Check sheet for the modelled part. Datum: model origin and axes. Units: mm. Round coordinates to 2 decimals unless told otherwise and drop trailing zeros. Write each loop counter-clockwise with the first axis right and the second up, starting at its lowest first coordinate (ties: lowest second). Pieces come first, ordered by that corner, then holes. Notation, with made-up numbers: (77.25, 41) -> (113.25, 41) arc R21 cw to (113.25, 70) -> close; hole circle Ø2 at (44.5, 52.5). An arc over 180 degrees is marked (long way). One line per item, written item: value.
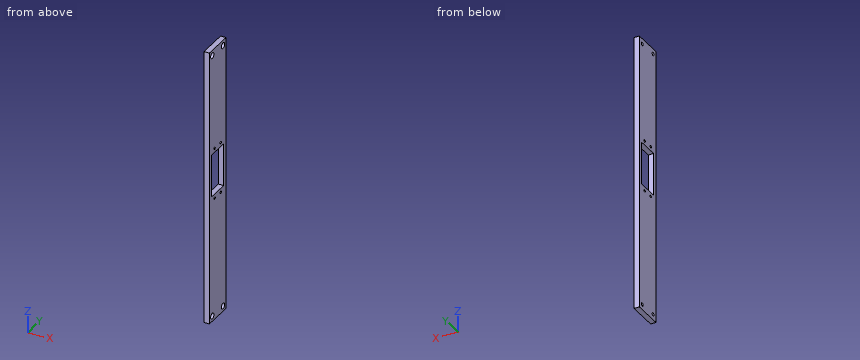
from build123d import *

# Parameters (mm, degrees)
SKETCH1_W                                  = 5
SKETCH1_H                                  = 260.2
BOSS_EXTRUDE1_DEPTH                        = 28
SKETCH2_W                                  = 40.12
SKETCH2_H                                  = 20.12
CUT_EXTRUDE1_DEPTH                         = 134.172857595
SKETCH3_R                                  = 1.125
CUT_EXTRUDE2_DEPTH                         = 134.172857595
SKETCH4_R                                  = 2.75
CUT_EXTRUDE3_DEPTH                         = 3
SKETCH5_R                                  = 1.55
CUT_EXTRUDE4_DEPTH                         = 134.112771739
MIRROR2_AT_THE_SECOND_PLANE_COPY_1_SKETC_R = 2.75
MIRROR2_AT_THE_SECOND_PLANE_COPY_1_DEPTH   = 3
MIRROR2_AT_THE_SECOND_PLANE_COPY_2_SKETC_R = 1.55
MIRROR2_AT_THE_SECOND_PLANE_COPY_2_DEPTH   = 134.112771739


with BuildPart() as part:
    # Sketch1 → Boss-Extrude1 (new body)
    with BuildSketch(Plane(origin=(0, 0, 0), x_dir=(1, 0, 0), z_dir=(0, 1, 0))):
        Rectangle(SKETCH1_W, SKETCH1_H)
    extrude(amount=BOSS_EXTRUDE1_DEPTH)

    # Sketch2 → Cut-Extrude1 (cut, through all)
    with BuildSketch(Plane(origin=(2.5, 0, 0), x_dir=(0, 0, -1), z_dir=(1, 0, 0))):
        with Locations((-10.06, 14)):
            Rectangle(SKETCH2_W, SKETCH2_H)
    extrude(amount=-CUT_EXTRUDE1_DEPTH, mode=Mode.SUBTRACT)

    # Sketch3 → Cut-Extrude2 (cut, through all)
    with BuildSketch(Plane(origin=(2.5, 0, 0), x_dir=(0, 0, -1), z_dir=(1, 0, 0))):
        with Locations((-33.96, 19.1)):
            Circle(SKETCH3_R)
        with Locations((-33.96, 8.9)):
            Circle(SKETCH3_R)
        with Locations((13.84, 19.1)):
            Circle(SKETCH3_R)
        with Locations((13.84, 8.9)):
            Circle(SKETCH3_R)
    extrude(amount=-CUT_EXTRUDE2_DEPTH, mode=Mode.SUBTRACT)

    # Sketch4 → Cut-Extrude3 (cut)
    with BuildSketch(Plane(origin=(2.5, 0, 0), x_dir=(0, 0, -1), z_dir=(1, 0, 0))):
        with Locations((-125.1, 23)):
            Circle(SKETCH4_R)
    cut_extrude3 = extrude(amount=-CUT_EXTRUDE3_DEPTH, mode=Mode.SUBTRACT)

    # Sketch5 → Cut-Extrude4 (cut, through all)
    with BuildSketch(Plane(origin=(-0.5, 0, 0), x_dir=(0, 0, -1), z_dir=(1, 0, 0))):
        with Locations((-125.1, 23)):
            Circle(SKETCH5_R)
    cut_extrude4 = extrude(amount=-CUT_EXTRUDE4_DEPTH, mode=Mode.SUBTRACT)

    # Mirror2: Cut-Extrude3, Cut-Extrude4 across plane
    add(cut_extrude3.mirror(Plane.XY), mode=Mode.SUBTRACT)
    add(cut_extrude4.mirror(Plane.XY), mode=Mode.SUBTRACT)

    # Mirror2 at the second plane: Cut-Extrude3, Cut-Extrude4 across plane
    add(cut_extrude3.mirror(Plane.ZX.offset(14)), mode=Mode.SUBTRACT)
    add(cut_extrude4.mirror(Plane.ZX.offset(14)), mode=Mode.SUBTRACT)

    # Mirror2 at the second plane copy 1 sketc → Mirror2 at the second plane copy 1 (cut)
    with BuildSketch(Plane(origin=(2.5, 28, 0), x_dir=(0, 0, 1), z_dir=(1, 0, 0))):
        with Locations((-125.1, 23)):
            Circle(MIRROR2_AT_THE_SECOND_PLANE_COPY_1_SKETC_R)
    extrude(amount=-MIRROR2_AT_THE_SECOND_PLANE_COPY_1_DEPTH, mode=Mode.SUBTRACT)

    # Mirror2 at the second plane copy 2 sketc → Mirror2 at the second plane copy 2 (cut, through all)
    with BuildSketch(Plane(origin=(-0.5, 28, 0), x_dir=(0, 0, 1), z_dir=(1, 0, 0))):
        with Locations((-125.1, 23)):
            Circle(MIRROR2_AT_THE_SECOND_PLANE_COPY_2_SKETC_R)
    extrude(amount=-MIRROR2_AT_THE_SECOND_PLANE_COPY_2_DEPTH, mode=Mode.SUBTRACT)


solid = part.part
Item 1: Sectioned sample at A-A (z = 3.5). Enter the section's corners in (x, y).
Result set:
outline: (-2.5, 0) -> (2.5, 0) -> (2.5, 3.94) -> (-2.5, 3.94) -> close; (-2.5, 24.06) -> (2.5, 24.06) -> (2.5, 28) -> (-2.5, 28) -> close
Item 2: Sectioned sample at B-B (y = 13). Enter the section's corners in (x, z), then the cut area to 3 significant figures.
Result set:
outline: (-2.5, -130.1) -> (2.5, -130.1) -> (2.5, -10) -> (-2.5, -10) -> close; (-2.5, 30.12) -> (2.5, 30.12) -> (2.5, 130.1) -> (-2.5, 130.1) -> close
area: 1,100 mm^2
Item 3: Depth check by flat-ended pin: pin 1 (2.5 mm diameter, centred on y = 5, z = 125.1, fed in from +X); pin 2 (4.5 mm diameter, centred on y = 22, z = 124, fed in from +X). Enter the tip coordinate at first touch or a pass-through.
Result set:
pin 1: through
pin 2: x = 2.5
Item 4: Sectioned sample at C-C (x = -1.45). State how many separate pieces and enclosed holes the cut face has, then the cut area to 3 significant figures.
Result set:
separate pieces: 1
enclosed holes: 9
area: 6,430 mm^2
Item 5: Material ranges on line 1 along Y through (x, z) = (1.1, -13.84) (3 decimals); line 2 along Z through (x, y) = (-1.5, 5); line 3 along Y through (x, z) = (-1.5, 125.1), recorded low to high.
Result set:
line 1: 0 to 7.775, 10.025 to 17.975, 20.225 to 28
line 2: -130.1 to -126.65, -123.55 to -10, 30.12 to 123.55, 126.65 to 130.1
line 3: 0 to 3.45, 6.55 to 21.45, 24.55 to 28
